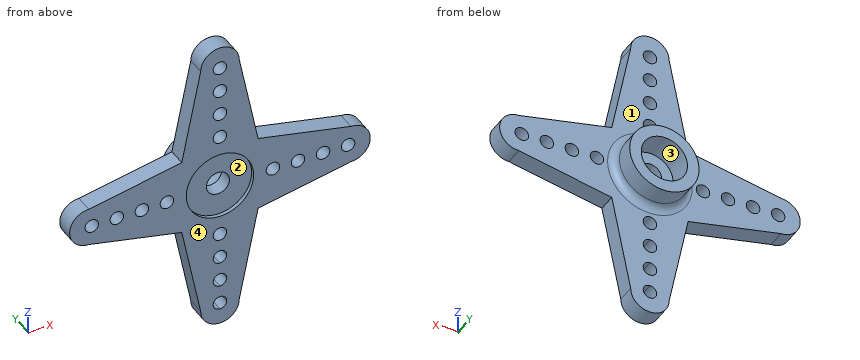
from build123d import *

# Parameters (mm, degrees)
SKETCH1_R           = 1.5
BOSS_EXTRUDE1_DEPTH = 2.4
SKETCH2_R           = 4.5
SKETCH2_R_2         = 3
BOSS_EXTRUDE2_DEPTH = 3.5
FILLET1_R           = 1
SKETCH3_R           = 0.875
CUT_EXTRUDE1_DEPTH  = 3.5
SKETCH4_R           = 4.375
CUT_EXTRUDE2_DEPTH  = 0.5


with BuildPart() as part:
    # Sketch1 → Boss-Extrude1 (new body)
    with BuildSketch(Plane(origin=(0, 0, 0), x_dir=(1, 0, 0), z_dir=(0, 1, 0))):
        with BuildLine():
            Line((-16.999165859, 2.5), (-4.949747468, 4.949747468))
            Line((-4.949747468, 4.949747468), (-2.5, 17.001645777))
            ThreePointArc((-2.5, 17.001645777), (0, 19.501645777), (2.5, 17.001645777))
            Line((2.5, 17.001645777), (4.949747468, 4.949747468))
            Line((4.949747468, 4.949747468), (17.000896169, 2.5))
            ThreePointArc((17.000896169, 2.5), (19.500896169, 0), (17.000896169, -2.5))
            Line((17.000896169, -2.5), (4.949747468, -4.949747468))
            Line((4.949747468, -4.949747468), (2.5, -16.999958072))
            ThreePointArc((2.5, -16.999958072), (0, -19.499958072), (-2.5, -16.999958072))
            Line((-2.5, -16.999958072), (-4.949747468, -4.949747468))
            Line((-4.949747468, -4.949747468), (-16.999165859, -2.5))
            ThreePointArc((-16.999165859, -2.5), (-19.499165859, 0), (-16.999165859, 2.5))
        make_face()
        Circle(SKETCH1_R, mode=Mode.SUBTRACT)
    extrude(amount=BOSS_EXTRUDE1_DEPTH)

    # Sketch2 → Boss-Extrude2 (add)
    with BuildSketch(Plane(origin=(0, 2.4, 0), x_dir=(1, 0, 0), z_dir=(0, 1, 0))):
        Circle(SKETCH2_R)
        Circle(SKETCH2_R_2, mode=Mode.SUBTRACT)
    extrude(amount=BOSS_EXTRUDE2_DEPTH)

    # Fillet1
    fillet1_edges = [part.edges().sort_by_distance(p)[0] for p in [
        (-4.5, 2.4, 0),
    ]]
    fillet(fillet1_edges, radius=FILLET1_R)

    # Sketch3 → Cut-Extrude1 (cut)
    with BuildSketch(Plane(origin=(0, 2.4, 0), x_dir=(1, 0, 0), z_dir=(0, 1, 0))):
        with Locations((0, -16.626645777)):
            Circle(SKETCH3_R)
        with Locations((0, -13.376645777)):
            Circle(SKETCH3_R)
        with Locations((0, -10.126645777)):
            Circle(SKETCH3_R)
        with Locations((0, -6.876645777)):
            Circle(SKETCH3_R)
        with Locations((-6.876645777, 0)):
            Circle(SKETCH3_R)
        with Locations((-10.126645777, 0)):
            Circle(SKETCH3_R)
        with Locations((-13.376645777, 0)):
            Circle(SKETCH3_R)
        with Locations((-16.626645777, 0)):
            Circle(SKETCH3_R)
        with Locations((0, 6.876645777)):
            Circle(SKETCH3_R)
        with BuildLine():
            ThreePointArc((0.875, 10.126645777), (0.618718434, 10.745364211), (0, 11.001645777))
            Line((0, 11.001645777), (0, 9.251645777))
            ThreePointArc((0, 9.251645777), (0.618718434, 9.507927344), (0.875, 10.126645777))
        make_face()
        with BuildLine():
            Line((0, 9.251645777), (0, 11.001645777))
            ThreePointArc((0, 11.001645777), (-0.875, 10.126645777), (0, 9.251645777))
        make_face()
        with BuildLine():
            ThreePointArc((0.875, 13.376645777), (0.618718434, 13.995364211), (0, 14.251645777))
            Line((0, 14.251645777), (0, 12.501645777))
            ThreePointArc((0, 12.501645777), (0.618718434, 12.757927344), (0.875, 13.376645777))
        make_face()
        with BuildLine():
            Line((0, 12.501645777), (0, 14.251645777))
            ThreePointArc((0, 14.251645777), (-0.875, 13.376645777), (0, 12.501645777))
        make_face()
        with BuildLine():
            ThreePointArc((0, 17.501645777), (-0.875, 16.626645777), (0, 15.751645777))
            Line((0, 15.751645777), (0, 17.501645777))
        make_face()
        with BuildLine():
            Line((0, 17.501645777), (0, 15.751645777))
            ThreePointArc((0, 15.751645777), (0.618718434, 16.007927344), (0.875, 16.626645777))
            ThreePointArc((0.875, 16.626645777), (0.618718434, 17.245364211), (0, 17.501645777))
        make_face()
        with Locations((6.876645777, 0)):
            Circle(SKETCH3_R)
        with Locations((13.376645777, 0)):
            Circle(SKETCH3_R)
        with Locations((16.626645777, 0)):
            Circle(SKETCH3_R)
        with Locations((10.126645777, 0)):
            Circle(SKETCH3_R)
    extrude(amount=-CUT_EXTRUDE1_DEPTH, mode=Mode.SUBTRACT)

    # Sketch4 → Cut-Extrude2 (cut)
    with BuildSketch(Plane.XZ):
        Circle(SKETCH4_R)
    extrude(amount=-CUT_EXTRUDE2_DEPTH, mode=Mode.SUBTRACT)


solid = part.part
Input: part model. Units: mm. Frame: model coordinates. Face numbers are marked on the shaded views. A direction names the side the tool comes from. Give positions to 0.01 mm unless a question says otherwise; leave off trailing zeros.
Q1. Pull-direction query (X, two-part tool) for the marked faces 3 and 4; classes: pulls with the +X half, pulls with the -X half, needs draft (parallel to the pull), parting line crosses it, or undercut.
Q2. Section A-A, the plane z = 0. State how many separate pieces and enclosed holes the cut face has, plus the area to 3 significant figures.
Q3. First-contact query: P1, Ø2, axis at x = 13.38, z = 0, coming from the -Y side; P2, Ø5, axis at x = 0, z = 0, coming from the -Y side; P3, Ø2.5, axis at x = 0, z = 16.63, coming from the +Y side. Flat tips, straight axial feed; report the tip coordinate or a pass-through.
Q4. Material intervals for probe 1 along Y at (x, z) = (5, 4); probe 2 along X at (y, z) = (2, -17); probe 3 along X at (y, z) = (1.65, 6.5), sorted ascending.
Q5. Set-up query: the marked faces 1 and 2. Return all of +Z, -Z, +X, -X, +Y, -Y with unobstructed straight access to the full face (end or side cutting, diameter ignored); none if empty.
Filled in:
1. face 3: undercut
1. face 4: needs draft
2. separate pieces: 10
2. enclosed holes: 0
2. area: 60.9 mm2
3. P1: stops at y = 0
3. P2: stops at y = 0.5
3. P3: stops at y = 2.4
4. probe 1: y = 0 to 2.4
4. probe 2: x = -2.5 to -0.79, 0.79 to 2.5
4. probe 3: x = -4.63 to -0.79, 0.79 to 4.63
5. face 1: +Y
5. face 2: -Y
